Can you work these out from the model? Positions are in its coordinate system, mm. Face numbers are marked on the shaded views. A direction names the side the tool comes from. Give positions to 0.01 mm unless a question says otherwise; leave off trailing zeros. Write each loop counter-clockwise with the first axis right and the second up, starting at its lowest first coordinate (ties: lowest second). Pieces come first, ordered by that corner, then holes.
```python
from build123d import *

# Parameters (mm, degrees)
SKETCH1_R               = 18.55
SKETCH1_R_2             = 3.55
BOSS_EXTRUDE1_DEPTH     = 2.56
SKETCH2_R               = 4.55
SKETCH2_R_2             = 3.55
BOSS_EXTRUDE2_DEPTH     = 20
SKETCH5_R               = 18.55
SKETCH5_R_2             = 3.55
BOSS_EXTRUDE3_DEPTH     = 2.56
SKETCH6_R               = 3.55
BOSS_EXTRUDE4_DEPTH     = 8
SKETCH7_R               = 1.5
CUT_EXTRUDE1_DEPTH      = 60.244741539
CUT_EXTRUDE1_DEPTH_BACK = 60.244741539


with BuildPart() as part:
    # Sketch1 → Boss-Extrude1 (new body)
    with BuildSketch(Plane(origin=(0, 0, 0), x_dir=(1, 0, 0), z_dir=(0, 1, 0))):
        with Locations(Location((0, 0, 0), (0, 0, 90))):
            Circle(SKETCH1_R)
        with Locations(Location((0, 0, 0), (0, 0, 90))):
            Circle(SKETCH1_R_2, mode=Mode.SUBTRACT)
    extrude(amount=BOSS_EXTRUDE1_DEPTH)

    # Sketch2 → Boss-Extrude2 (add)
    with BuildSketch(Plane(origin=(0, 2.56, 0), x_dir=(1, 0, 0), z_dir=(0, 1, 0))):
        with Locations(Location((0, 0, 0), (0, 0, 270))):
            Circle(SKETCH2_R)
        with Locations(Location((0, 0, 0), (0, 0, 90))):
            Circle(SKETCH2_R_2, mode=Mode.SUBTRACT)
    boss_extrude2 = extrude(amount=BOSS_EXTRUDE2_DEPTH)

    # Mirror1: Boss-Extrude2 across plane
    add(boss_extrude2.mirror(Plane.ZX.offset(22.56)))

    # Sketch5 → Boss-Extrude3 (add)
    with BuildSketch(Plane(origin=(0, 42.56, 0), x_dir=(1, 0, 0), z_dir=(0, 1, 0))):
        with Locations(Location((0, 0, 0), (0, 0, 90))):
            Circle(SKETCH5_R)
        with Locations(Location((0, 0, 0), (0, 0, 90))):
            Circle(SKETCH5_R_2, mode=Mode.SUBTRACT)
    extrude(amount=BOSS_EXTRUDE3_DEPTH)

    # Sketch6 → Boss-Extrude4 (add)
    with BuildSketch(Plane(origin=(0, 45.12, 0), x_dir=(1, 0, 0), z_dir=(0, 1, 0))):
        Polygon((-5.794958779, 0), (-2.897479389, -5.018581516), (2.897479389, -5.018581516), (5.794958779, 0), (2.897479389, 5.018581516), (-2.897479389, 5.018581516), align=None)
        with Locations(Location((0, 0, 0), (0, 0, 90))):
            Circle(SKETCH6_R, mode=Mode.SUBTRACT)
    extrude(amount=BOSS_EXTRUDE4_DEPTH)

    # Sketch7 → Cut-Extrude1 (cut, two sides)
    with BuildSketch(Plane.XZ) as cut_extrude1_sk:
        with Locations(Location((-13.371154887, -3, 0), (0, 0, 270))):
            Circle(SKETCH7_R)
        with Locations(Location((-13.371154887, 3, 0), (0, 0, 270))):
            Circle(SKETCH7_R)
    extrude(amount=CUT_EXTRUDE1_DEPTH, mode=Mode.SUBTRACT)
    extrude(cut_extrude1_sk.sketch, amount=-CUT_EXTRUDE1_DEPTH_BACK, mode=Mode.SUBTRACT)


solid = part.part
```
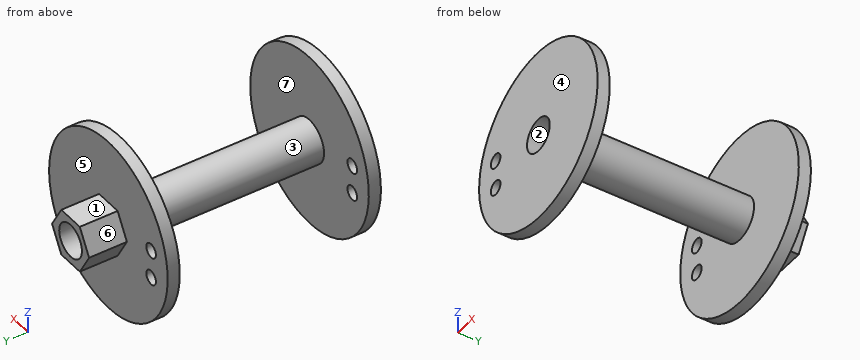
1) Suppose I cut it at B-B on z = -12.5. Write out the boundary of the cut face in (x, y).
Values follow:
outline: (-13.71, 0) - (13.71, 0) - (13.71, 2.56) - (-13.71, 2.56) - close; (-13.71, 42.56) - (13.71, 42.56) - (13.71, 45.12) - (-13.71, 45.12) - close
2) For the marked faces 1, 2 and 3, which set-ups out of +Z, -Z, +X, -X, +Y, -Y let a thin tool reach every point of the face, with its end or its side?
Values follow:
face 1: +Z, +X, -X, +Y
face 2: +Y, -Y
face 3: none
3) Suppose I cut it at D-D on y = 24. Write out the boundary of the cut face in (x, z).
Values follow:
outline: circle Ø9.1 at (0, 0); hole circle Ø7.1 at (0, 0)
4) Please list where these lines run through material, in increasing order: L1, parallel to X at y = 35.5, z = 0; L2, parallel to Y at x = -2, z = 17; L3, parallel to X at y = 43.3, z = 3.
Values follow:
L1: x = -4.55 to -3.55, 3.55 to 4.55
L2: y = 0 to 2.56, 42.56 to 45.12
L3: x = -18.31 to -14.87, -11.87 to -1.9, 1.9 to 18.31
5) If we mould it in two halves opening along Y, with no side actions, what happens to the marked faces 4, 5, 6 and 7? For each: +Y half, -Y half, draft (parallel to the pull), parting line (faces both ways), or undercut.
Values follow:
face 4: -Y half
face 5: +Y half
face 6: draft
face 7: undercut
6) For pin 1 Ø10 at (y, z) = (28.5, 4.5) entering from +X; pin 2 Ø1.8 at (x, z) = (-13.37, -3) entering from +Y; pin 3 Ø12 at (y, z) = (7, 1.5) entering from +X; pin 4 Ø4 at (x, y) = (4.5, 24.5) entering from +Z, each with a flat end and sliding along its axis, tell me the tip position at first contact or that it passes through.
Values follow:
pin 1: stops at x = 4.55
pin 2: passes through
pin 3: stops at x = 18.55
pin 4: stops at z = 3.8
7) Suppose I cut it at A-A on x = 0. Write out the boundary of the cut face in (y, z).
Values follow:
outline: (0, -18.55) - (2.56, -18.55) - (2.56, -4.55) - (42.56, -4.55) - (42.56, -18.55) - (45.12, -18.55) - (45.12, -5.02) - (53.12, -5.02) - (53.12, -3.55) - (0, -3.55) - close; (0, 3.55) - (53.12, 3.55) - (53.12, 5.02) - (45.12, 5.02) - (45.12, 18.55) - (42.56, 18.55) - (42.56, 4.55) - (2.56, 4.55) - (2.56, 18.55) - (0, 18.55) - close
8) Suppose I cut it at C-C on x = 11. Write out the boundary of the cut face in (y, z).
Values follow:
outline: (0, -14.94) - (2.56, -14.94) - (2.56, 14.94) - (0, 14.94) - close; (42.56, -14.94) - (45.12, -14.94) - (45.12, 14.94) - (42.56, 14.94) - close
